```python
from build123d import *

# Parameters (mm, degrees)
F1_DEPTH = 2.794
F5_DEPTH = 25.4


# Not quite as in the source:
# - a feature of the source that left no trace in its solid (it failed there, or was rolled back) is left out
# - the program builds the solid bodies; features that only make, move or delete a surface that nothing else refers to are left out


with BuildPart() as f1:
    # F0 (on Top) → F1 (new body)
    with BuildSketch(Plane.XY):
        with BuildLine():
            Line((-16.4724217036, 22.0521983965), (-40.4838242176, 22.0521983965))
            Line((-40.4838242176, 22.0521983965), (-40.4838242176, -9.8933519139))
            ThreePointArc((-40.4838242176, -9.8933519139), (-40.4370025072, -9.928574703), (-40.3900778613, -9.963660242))
            Line((-40.3900778613, -9.963660242), (-16.4724217036, -9.963660242))
            Line((-16.4724217036, -9.963660242), (-16.4724217036, 22.0521983965))
        make_face()
    extrude(amount=F1_DEPTH)

    # F0 (on Top) → F5 (join)
    with BuildSketch(Plane.XY):
        with BuildLine():
            Line((-40.4838242176, -9.8933519139), (-40.4838242176, 22.0521983965))
            ThreePointArc((-40.4838242176, 22.0521983965), (-48.4410997737, 6.0794232413), (-40.4838242176, -9.8933519139))
        make_face()
    extrude(amount=F5_DEPTH)


solid = f1.part
```
The model under review builds one solid part; all positions refer to its coordinate system, in mm. A direction names the side the tool comes from. Give positions to 0.01 mm unless a question says otherwise; leave off trailing zeros. Write each loop counter-clockwise with the first axis right and the second up, starting at its lowest first coordinate (ties: lowest second). Pieces come first, ordered by that corner, then holes. Notation, with made-up numbers: M -2.75,77.5 L 30.25,77.5 A28 ccw 30.25,108.5 Z; hole C 41.25,5.25 d6. An arc over 180 degrees is marked long. Write each question's results on one line, items separated by ' | '. Start each with the question number.
1. We need section D-D (y = -5.5). Write out the cut boundary in (x, z), and give its area (3 significant figures).
2. We need section A-A (y = 1). Write out the cut boundary in (x, z), and give its area (3 significant figures).
3. We need section C-C (z = 3.75). Write out the cut boundary in (x, y), and give its area (3 significant figures).
4. For probe 1 along Z at (x, y) = (-34.5, 7.5); probe 2 along X at (y, z) = (4, 8); probe 3 along X at (y, z) = (-4, 3.5), list the stretches that pass through material, from the lowest coordinate up. Write a range as [from, to].
5. For faces 1 (the flat face through (-28, 22.052, 1)), 2 (the flat face through (-29, 6, 2.794)), list the 3-axis set-ups (+Z, -Z, +X, -X, +Y, -Y) from which the entire face can be reached by the end or side of a thin tool; tool diameter is ignored.
6. Insertion check: pin 1 Ø2 at (y, z) = (18.5, 3) entering from -X; pin 2 Ø8 at (y, z) = (9, 13.5) entering from -X; pin 3 Ø8 at (y, z) = (-1.5, 12.5) entering from -X; pin 4 Ø1 at (x, y) = (-28.5, -6) entering from +Z. Each pin has a flat end and moves straight along its axis. Give the tip position at first contact, or say it passes through.
7. We need section B-B (x = -37). Write out the cut boundary in (y, z).
Results found:
1) outline: M -44.75,0 L -16.47,0 L -16.47,2.79 L -40.48,2.79 L -40.48,25.4 L -44.75,25.4 Z | area: 175 mm^2
2) outline: M -47.79,0 L -16.47,0 L -16.47,2.79 L -40.48,2.79 L -40.48,25.4 L -47.79,25.4 Z | area: 253 mm^2
3) outline: M -40.48,-9.89 L -40.48,22.05 A20.01 ccw Z | area: 178 mm^2
4) probe 1: z = [0, 2.79] | probe 2: x = [-48.33, -40.48] | probe 3: x = [-45.72, -40.48]
5) face 1: +Z, -Z, +X, -X, +Y | face 2: +Z, +X, +Y, -Y
6) pin 1: stops at x = -44.86 | pin 2: stops at x = -48.44 | pin 3: stops at x = -48.12 | pin 4: stops at z = 2.79
7) outline: M -9.96,0 L 22.05,0 L 22.05,2.79 L -9.96,2.79 Z
